Could you check a few things on this model? Use its own coordinates, in mm. A direction names the side the tool comes from. Give positions to 0.01 mm unless a question says otherwise; leave off trailing zeros. Order: outer loops, then holes, each group sorted by start corner. A loop starts at its lowest first (then second) coordinate and runs counter-clockwise, first axis right, second up. Notation, with made-up numbers: (17.5, -32.75) - (34.5, -32.75) arc R21 cw to (34.5, -3.75) - close; hole circle Ø3 at (32, -25.75). An arc over 180 degrees is marked (long way). Put each result on its own line as item: value.
Autodesk Inventor part; units mm, degrees
ref_plane "YZ Plane" through (0, 0, 0) normal (1, 0, 0) x (0, 1, 0)
ref_plane "XZ Plane" through (0, 0, 0) normal (0, 1, 0) x (-1, 0, 0)
ref_plane "XY Plane" through (0, 0, 0) normal (0, 0, 1) x (1, 0, 0)
sketch "Esquisse1" plane through (0, 0, 0) normal (0, 0, 1) x (1, 0, 0)
  line L0 (0, 0) -> (20, 0)
  line L1 (20, 0) -> (20, 16)
  line L2 (20, 16) -> (0, 16)
  line L3 (0, 16) -> (0, 0)
  dimension "d0" = 20
  dimension "d1" = 16
extrude "Extrusion1" add sketch "Esquisse1" along normal blind 3
sketch "Esquisse2" plane through (0, 0, 3) normal (0, 0, 1) x (1, 0, 0)
  line L0 (20, 0) -> (20, 16)
  line L1 (20, 8) -> (0, 8)
  line L2 (0, 16) -> (0, 0)
  line L3 (20, 16) -> (0, 16)
  line L4 (0, 16) -> (0, 14)
  line L5 (0, 14) -> (20, 14)
  line L6 (20, 14) -> (20, 16)
  line L7 (20, 16) -> (19.25, 16)
  line L8 (19.25, 16) -> (19.25, 14)
  line L9 (19.25, 14) -> (20, 14)
  line L10 (20, 14) -> (20, 16)
  line L11 (19.25, 14) -> (17.25, 14)
  line L12 (17.25, 14) -> (17.25, 16)
  line L13 (17.25, 16) -> (16.5, 16)
  line L14 (16.5, 16) -> (16.5, 14)
  line L15 (16.5, 14) -> (17.25, 14)
  line L16 (17.25, 14) -> (17.25, 16)
  line L17 (16.5, 14) -> (14.5, 14)
  line L18 (14.5, 14) -> (14.5, 16)
  line L19 (14.5, 16) -> (13.75, 16)
  line L20 (13.75, 16) -> (13.75, 14)
  line L21 (13.75, 14) -> (14.5, 14)
  line L22 (14.5, 14) -> (14.5, 16)
  line L23 (13.75, 14) -> (11.75, 14)
  line L24 (11.75, 14) -> (11.75, 16)
  line L25 (11.75, 16) -> (11, 16)
  line L26 (11, 16) -> (11, 14)
  line L27 (11, 14) -> (11.75, 14)
  line L28 (11.75, 14) -> (11.75, 16)
  line L29 (11, 14) -> (9, 14)
  line L30 (9, 14) -> (9, 16)
  line L31 (9, 16) -> (8.25, 16)
  line L32 (8.25, 16) -> (8.25, 14)
  line L33 (8.25, 14) -> (9, 14)
  line L34 (9, 14) -> (9, 16)
  line L35 (8.25, 14) -> (6.25, 14)
  line L36 (6.25, 14) -> (6.25, 16)
  line L37 (6.25, 16) -> (5.5, 16)
  line L38 (5.5, 16) -> (5.5, 14)
  line L39 (5.5, 14) -> (6.25, 14)
  line L40 (6.25, 14) -> (6.25, 16)
  line L41 (5.5, 14) -> (3.5, 14)
  line L42 (3.5, 14) -> (3.5, 16)
  line L43 (3.5, 16) -> (2.75, 16)
  line L44 (2.75, 16) -> (2.75, 14)
  line L45 (2.75, 14) -> (3.5, 14)
  line L46 (3.5, 14) -> (3.5, 16)
  line L47 (2.75, 14) -> (0.75, 14)
  line L48 (0.75, 14) -> (0.75, 16)
  line L49 (20, 0) -> (0, 0)
  line L50 (0, 0) -> (0, 2)
  line L51 (0, 2) -> (20, 2)
  line L52 (20, 2) -> (20, 0)
  line L53 (20, 0) -> (19.25, 0)
  line L54 (19.25, 0) -> (19.25, 2)
  line L55 (19.25, 2) -> (20, 2)
  line L56 (20, 2) -> (20, 0)
  line L57 (19.25, 2) -> (17.25, 2)
  line L58 (17.25, 2) -> (17.25, 0)
  line L59 (17.25, 0) -> (16.5, 0)
  line L60 (16.5, 0) -> (16.5, 2)
  line L61 (16.5, 2) -> (17.25, 2)
  line L62 (17.25, 2) -> (17.25, 0)
  line L63 (16.5, 2) -> (14.5, 2)
  line L64 (14.5, 2) -> (14.5, 0)
  line L65 (14.5, 0) -> (13.75, 0)
  line L66 (13.75, 0) -> (13.75, 2)
  line L67 (13.75, 2) -> (14.5, 2)
  line L68 (14.5, 2) -> (14.5, 0)
  line L69 (13.75, 2) -> (11.75, 2)
  line L70 (11.75, 2) -> (11.75, 0)
  line L71 (11.75, 0) -> (11, 0)
  line L72 (11, 0) -> (11, 2)
  line L73 (11, 2) -> (11.75, 2)
  line L74 (11.75, 2) -> (11.75, 0)
  line L75 (11, 2) -> (9, 2)
  line L76 (9, 2) -> (9, 0)
  line L77 (9, 0) -> (8.25, 0)
  line L78 (8.25, 0) -> (8.25, 2)
  line L79 (8.25, 2) -> (9, 2)
  line L80 (9, 2) -> (9, 0)
  line L81 (8.25, 2) -> (6.25, 2)
  line L82 (6.25, 2) -> (6.25, 0)
  line L83 (6.25, 0) -> (5.5, 0)
  line L84 (5.5, 0) -> (5.5, 2)
  line L85 (5.5, 2) -> (6.25, 2)
  line L86 (6.25, 2) -> (6.25, 0)
  line L87 (5.5, 2) -> (3.5, 2)
  line L88 (3.5, 2) -> (3.5, 0)
  line L89 (3.5, 0) -> (2.75, 0)
  line L90 (2.75, 0) -> (2.75, 2)
  line L91 (2.75, 2) -> (3.5, 2)
  line L92 (3.5, 2) -> (3.5, 0)
  line L93 (2.75, 2) -> (0.75, 2)
  line L94 (0.75, 2) -> (0.75, 0)
  point P0 (0, 0)
  dimension "d4" = 2
  dimension "d5" = 0.75
  dimension "d6" = 2
  dimension "d7" = 2
  dimension "d8" = 2
  dimension "d9" = 2
  dimension "d10" = 2
  dimension "d11" = 2
  dimension "d12" = 2
extrude "Extrusion2" add sketch "Esquisse2" along normal blind 4 contours L49 L54 L51 L0 | L49 L60 L51 L58 | L5 L8 L3 L0 | L2 L3 L48 L5 | L51 L94 L49 L2 | L49 L66 L51 L64 | L5 L14 L3 L12 | L44 L3 L42 L5 | L51 L88 L49 L90 | L49 L72 L51 L70 | L5 L20 L3 L18 | L38 L3 L36 L5 | L51 L82 L49 L84 | L49 L78 L51 L76 | L5 L26 L3 L24 | L32 L3 L30 L5
properties part number "driver DRV8825"
1) Suppose I cut it at B-B, the plane z = 6.75. State how many separate pieces and enclosed holes the cut face has, and give its area (3 significant figures).
Filled in:
separate pieces: 16
enclosed holes: 0
area: 24.0 mm^2
2) I'm going to push a flat-ended pin straight in: pin 1 (1.5 mm diameter, centred on x = 5, y = 7.5, fed in from +Z). Where does the tip first touch, or does it pass through?
Filled in:
pin 1: stops at z = 3
3) We'd pull the mould along X, two halves only. Please class faces 1 (the flat face through (20, 8, 2)), 2 (the flat face through (9, 15, 5)), 3 (the flat face through (9.9, 0, 2.7)), 4 (the flat face through (11, 1, 5)): pulls with the +X half, pulls with the -X half, needs draft (parallel to the pull), parting line crosses it, or undercut.
Filled in:
face 1: pulls with the +X half
face 2: undercut
face 3: needs draft
face 4: undercut
4) Suppose I cut it at C-C, the plane y = 7.25. List the corners of the cut face in (x, z) for me, and give its area (3 significant figures).
Filled in:
outline: (0, 0) - (20, 0) - (20, 3) - (0, 3) - close
area: 60.0 mm^2
5) Which directions (+Z, -Z, +X, -X, +Y, -Y) give clear straight access to the entire face, cutting with the end or side of a thin tool? Please do faces 5 (the flat face through (10, 8, 0)), 6 (the flat face through (16.5, 1, 5)).
Filled in:
face 5: -Z, +X, -X, +Y, -Y
face 6: +Z, +Y, -Y
6) Suppose I cut it at D-D, the plane x = 1.75. List the corners of the cut face in (y, z) for me, and give its area (3 significant figures).
Filled in:
outline: (0, 0) - (16, 0) - (16, 3) - (0, 3) - close
area: 48.0 mm^2
7) If I drill on line 1 (Z direction, x = 6, y = 11.5); line 2 (Y direction, x = 5.75, z = 6), over which ranges is the centre line in solid material (lowest first)? Write a range as [from, to].
Filled in:
line 1: z = [0, 3]
line 2: y = [0, 2], [14, 16]
8) Suppose I cut it at A-A, the plane x = 16.75. List the corners of the cut face in (y, z) for me.
Filled in:
outline: (0, 0) - (16, 0) - (16, 7) - (14, 7) - (14, 3) - (2, 3) - (2, 7) - (0, 7) - close
